The listing builds one solid part. Answer for the finished solid, in the listing's coordinates (mm). Round coordinates to 2 decimals unless told otherwise and drop trailing zeros. Write each loop counter-clockwise with the first axis right and the second up, starting at its lowest first coordinate (ties: lowest second). Pieces come first, ordered by that corner, then holes. Notation, with made-up numbers: (-34.75, 15.25) - (17.25, 15.25) arc R18 cw to (17.25, 20.25) - close; hole circle Ø8 at (53.25, 49). An arc over 180 degrees is marked (long way). Answer as CSV lines item,"result". Start each with the question number.
Item 1: A cutting plane is placed at A-A on x = 0. Determine the outline of the cut face in (y, z), and give its area (3 significant figures).
Item 2: A cutting plane is placed at D-D on y = 132.5. Determine the outline of the cut face in (x, z).
Item 3: A cutting plane is placed at B-B on z = 0. Determine the outline of the cut face in (x, y).
Item 4: Flat-ended cylindrical pins translate along their axes: pin 1 (8 mm diameter, centred on x = -238.5, y = 83, fed in from -Z); pin 2 (2 mm diameter, centred on y = 125, z = -400.5, fed in from +X); pin 3 (6 mm diameter, centred on x = 280, z = -711.5, fed in from +Y). Find the tip coordinate at first contact, or state that the pin passes through.
Item 5: Straight lines are drawn through the part: line 1 along Z through (x, y) = (0, 23); line 2 along X through (y, z) = (119, 767); line 3 along X through (y, z) = (218.5, -376). For each, find the intervals that lie inside material, in ascending order. Write a range as [from, to].
Item 6: For a pull along X with two mould halves and no side action, classify faces 1 (the cylindrical face through (858.44, 22.82, -270.34)), 2 (the flat face through (-662, 0, 596)), 3 (the cylindrical face through (846.994, 22.185, -266.731)) as pulls with the +X half, pulls with the -X half, needs draft (parallel to the pull), parting line crosses it, or undercut.
```python
from build123d import *


with BuildPart() as part:
    # Rotationsschnitt → Klöpperboden (revolve)
    with BuildSketch(Plane.XY, mode=Mode.PRIVATE) as kl_pperboden_sk:
        with BuildLine():
            Line((-900, 0), (-900, 45))
            ThreePointArc((-900, 45), (-870.766611209, 146.810039133), (-791.972993744, 217.601570654))
            ThreePointArc((-791.972993744, 217.601570654), (-406.334858199, 353.692763685), (0, 399.84))
            Line((0, 399.84), (0, 387.84))
            ThreePointArc((0, 387.84), (-403.643898873, 341.998374521), (-786.72813948, 206.80844767))
            ThreePointArc((-786.72813948, 206.80844767), (-860.594633743, 140.443652841), (-888, 45))
            Line((-888, 45), (-888, 0))
            Line((-888, 0), (-900, 0))
        make_face()
    revolve(kl_pperboden_sk.sketch.rotate(Axis((0, 0, 0), (0, 1, 0)), 180), axis=Axis((0, 0, 0), (0, 1, 0)))  # turned: the seam where the file's is


solid = part.part
```
Geometry says:
1,outline,"(0, -900) - (45, -900) arc R191.9 ccw to (217.6, -791.97) arc R1812 ccw to (217.6, 791.97) arc R191.9 ccw to (45, 900) - (0, 900) - (0, 888) - (45, 888) arc R179.9 cw to (206.81, 786.73) arc R1800 cw to (206.81, -786.73) arc R179.9 cw to (45, -888) - (0, -888) - close"
1,area,"25,700 mm^2"
2,outline,"circle Ø1757.78 at (0, 0); hole circle Ø1730.57 at (0, 0)"
3,outline,"(-900, 0) - (-888, 0) - (-888, 45) arc R179.9 cw to (-786.73, 206.81) arc R1800 cw to (786.73, 206.81) arc R179.9 cw to (888, 45) - (888, 0) - (900, 0) - (900, 45) arc R191.9 ccw to (791.97, 217.6) arc R1812 ccw to (-791.97, 217.6) arc R191.9 ccw to (-900, 45) - close"
4,pin 1,"stops at z = -865.25"
4,pin 2,"stops at x = 787.14"
4,pin 3,"stops at y = 232.01"
5,line 1,"z = [-900, -888], [888, 900]"
5,line 2,"x = [-441.83, -415], [415, 441.83]"
5,line 3,"x = [-694.92, -663], [663, 694.92]"
6,face 1,"parting line crosses it"
6,face 2,"needs draft"
6,face 3,"undercut"
